CAD build for the part. Positions are in the model's coordinates, mm. Face numbers are marked on the shaded views. A direction names the side the tool comes from. Round coordinates to 2 decimals unless told otherwise and drop trailing zeros. Loops run counter-clockwise (first coordinate to the right, second up) from the corner with the lowest first, then second, coordinate; pieces in that order, holes last. Notation, with made-up numbers: M 31,58.5 L 36,58.5 A22 ccw 36,95.5 Z; hole C 81.25,-1 d3. An arc over 180 degrees is marked long. Use one line per item in the form item = value.
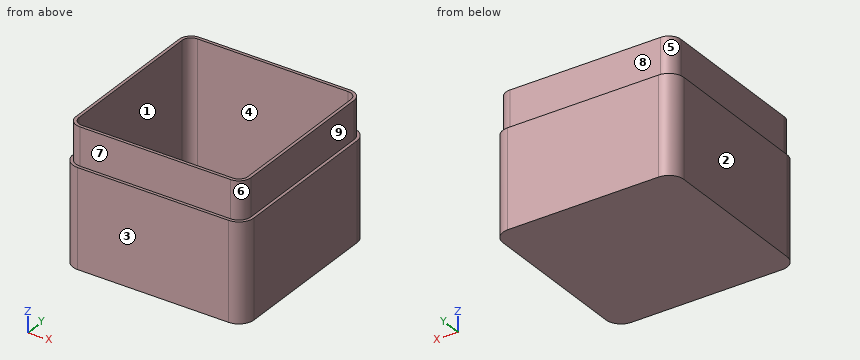
from build123d import *

# Parameters (mm, degrees)
CROQUIS1_W              = 120
CROQUIS1_H              = 120
SALIENTE_EXTRUIR1_DEPTH = 90
REDONDEO2_R             = 10
VACIADO1_T              = -4
CROQUIS6_OUTSIDE_W      = 160.418
CROQUIS6_OUTSIDE_H      = 160.418
CORTAR_EXTRUIR2_DEPTH   = 25


with BuildPart() as part:
    # Croquis1 → Saliente-Extruir1 (new body)
    with BuildSketch(Plane.XY):
        with Locations((60, 60)):
            Rectangle(CROQUIS1_W, CROQUIS1_H)
    extrude(amount=SALIENTE_EXTRUIR1_DEPTH)

    # Redondeo2
    redondeo2_edges = [part.edges().sort_by_distance(p)[0] for p in [
        (0, 120, 45),
        (120, 120, 45),
        (120, 0, 45),
        (0, 0, 45),
    ]]
    fillet(redondeo2_edges, radius=REDONDEO2_R)

    # Vaciado1
    vaciado1_openings = [part.faces().sort_by_distance(p)[0] for p in [
        (60, 60, 90),
    ]]
    offset(amount=VACIADO1_T, openings=vaciado1_openings, kind=Kind.INTERSECTION)

    # Croquis6 outside → Cortar-Extruir2 (cut)
    with BuildSketch(Plane.XY.offset(90)):
        with Locations((60, 60)):
            Rectangle(CROQUIS6_OUTSIDE_W, CROQUIS6_OUTSIDE_H)
        with BuildLine():
            Line((10, 2), (110, 2))
            ThreePointArc((110, 2), (115.656854249, 4.343145751), (118, 10))
            Line((118, 10), (118, 110))
            ThreePointArc((118, 110), (115.656854249, 115.656854249), (110, 118))
            Line((110, 118), (10, 118))
            ThreePointArc((10, 118), (4.343145751, 115.656854249), (2, 110))
            Line((2, 110), (2, 10))
            ThreePointArc((2, 10), (4.343145751, 4.343145751), (10, 2))
        make_face(mode=Mode.SUBTRACT)
    extrude(amount=-CORTAR_EXTRUIR2_DEPTH, mode=Mode.SUBTRACT)


solid = part.part
1. Cut at B-B on y = 30. Write the cut outline in (x, z).
Completed:
outline = M 0,0 L 120,0 L 120,65 L 118,65 L 118,90 L 116,90 L 116,4 L 4,4 L 4,90 L 2,90 L 2,65 L 0,65 Z
2. Cut at D-D on z = 32.5. Write the cut outline in (x, y), and give its area (3 significant figures).
Completed:
outline = M 0,10 A10 ccw 10,0 L 110,0 A10 ccw 120,10 L 120,110 A10 ccw 110,120 L 10,120 A10 ccw 0,110 Z; hole M 4,10 A6 ccw 10,4 L 110,4 A6 ccw 116,10 L 116,110 A6 ccw 110,116 L 10,116 A6 ccw 4,110 Z
area = 1,800 mm2
3. Cut at A-A on z = 73. Write the cut outline in (x, y).
Completed:
outline = M 2,10 A8 ccw 10,2 L 110,2 A8 ccw 118,10 L 118,110 A8 ccw 110,118 L 10,118 A8 ccw 2,110 Z; hole M 4,10 A6 ccw 10,4 L 110,4 A6 ccw 116,10 L 116,110 A6 ccw 110,116 L 10,116 A6 ccw 4,110 Z
4. Pull direction Y, two halves, no side cores. Call the marked faces 1, 2, 3 and 4: +Y half, -Y half, draft (parallel to the pull), parting line (faces both ways), or undercut.
Completed:
face_1 = undercut
face_2 = draft
face_3 = -Y half
face_4 = undercut
5. Tool access for the marked faces 5, 6, 7, 8 and 9: list every direction of +Z, -Z, +X, -X, +Y, -Y with a clear straight run to the whole face (end or side of a thin tool).
Completed:
face_5 = +Z, -X, +Y
face_6 = +Z, +X, -Y
face_7 = +Z, +X, -X, -Y
face_8 = +Z, +X, -X, +Y
face_9 = +Z, +X, +Y, -Y
6. Probe line 1 along X through (y, z) = (22, 46.5); line 2 along Y through (x, z) = (10, 68.5). List the from-to ranges inside material, lowest first. Write a range as from..to.
Completed:
line_1 = 0..4, 116..120
line_2 = 2..4, 116..118
7. Drop flat-ended pins along their axis: P1, Ø20, axis at x = 74, z = 78, coming from the +Y side; P2, Ø6, axis at x = 83, y = 39.5, coming from the +Z side; P3, Ø2, axis at x = 54, z = 67, coming from the -Y side. Give the stop position or say it passes through.
Completed:
P1 = 118
P2 = 4
P3 = 2
